Autodesk Inventor part; units mm, degrees
ref_plane "YZ Plane" through (0, 0, 0) normal (1, 0, 0) x (0, 1, 0)
ref_plane "XZ Plane" through (0, 0, 0) normal (0, 1, 0) x (-1, 0, 0)
ref_plane "XY Plane" through (0, 0, 0) normal (0, 0, 1) x (1, 0, 0)
sketch "Sketch1" plane through (0, 0, 0) normal (0, 0, 1) x (1, 0, 0)
  line L0 (-26.924, 25.4) -> (26.924, 25.4)
  line L1 (-26.924, 25.4) -> (-26.924, -19.05)
  line L2 (-14.224, -25.4) -> (-14.224, -20.32)
  line L3 (-15.494, -19.05) -> (-26.924, -19.05)
  line L4 (26.924, 25.4) -> (26.924, -19.05)
  line L5 (26.924, -19.05) -> (15.494, -19.05)
  line L6 (14.224, -20.32) -> (14.224, -25.4)
  line L7 (14.224, -25.4) -> (-14.224, -25.4)
  line L8 (-15.494, -19.05) -> (-14.224, -20.32)
  line L9 (14.224, -20.32) -> (15.494, -19.05)
  point P0 (0, 0)
  point P1 (-14.224, -19.05)
  point P2 (14.224, -19.05)
  dimension "d7" = 1.27
  dimension "d8" = 1.27
  dimension "d9" = 1.27
  dimension "d10" = 1.27
extrude "Extrusion1" add sketch "Sketch1" along normal blind 1.6
sketch "Sketch2" plane through (0, 0, 1.6) normal (0, 0, 1) x (1, 0, 0)
  line L0 (26.924, 25.4) -> (-26.924, 25.4)
  line L1 (-26.924, 25.4) -> (-26.924, 22.225)
  line L2 (-26.924, 25.4) -> (-26.924, -19.05)
  line L3 (-26.924, 22.225) -> (-23.749, 22.225)
  line L4 (26.924, 22.225) -> (23.749, 22.225)
  line L5 (14.224, -25.4) -> (-14.224, -25.4)
  line L6 (-14.224, -25.4) -> (-11.049, -25.4)
  line L7 (-11.049, -25.4) -> (-11.049, -22.225)
  line L8 (14.224, -25.4) -> (11.049, -25.4)
  line L9 (11.049, -25.4) -> (11.049, -22.225)
  line L10 (-26.924, -19.05) -> (-26.924, -10.922)
  line L11 (-26.924, -10.922) -> (-23.749, -10.922)
  point P0 (0, 0)
  dimension "d13" = 3.175
  dimension "d14" = 3.175
  dimension "d15" = 3.175
  dimension "d16" = 3.175
  dimension "d17" = 3.175
  dimension "d18" = 3.175
  dimension "d19" = 8.128
  dimension "d20" = 3.175
hole "Hole1" at (-23.749, 22.225, 1.6) at (23.749, 22.225, 1.6) at (-11.049, -22.225, 1.6) at (11.049, -22.225, 1.6) at (-23.749, -10.922, 1.6) direction (0, 0, -1) diameter 3.048 end through all
sketch "Sketch3" plane through (0, 0, 1.6) normal (0, 0, 1) x (1, 0, 0)
  line L0 (-26.924, 25.4) -> (26.924, 25.4)
  line L1 (0, 23.4) -> (8.5, 23.4)
  line L2 (8.5, 23.4) -> (8.5, 16.9)
  line L3 (8.5, 6.4) -> (-8.5, 6.4)
  line L4 (-8.5, 6.4) -> (-8.5, 12.9)
  line L5 (-8.5, 23.4) -> (0, 23.4)
  line L6 (-8.5, 23.4) -> (-8.5, 16.9)
  line L7 (-8.5, 12.9) -> (-10.5, 12.9)
  line L8 (-12.5, 14.9) -> (-12.5, 14.9)
  line L9 (-10.5, 16.9) -> (-8.5, 16.9)
  line L10 (-8.5, 16.9) -> (-8.5, 23.4)
  line L11 (8.5, 12.9) -> (10.5, 12.9)
  line L12 (12.5, 14.9) -> (12.5, 14.9)
  line L13 (10.5, 16.9) -> (8.5, 16.9)
  line L14 (8.5, 12.9) -> (8.5, 6.4)
  arc A0 (-10.5, 16.9) -> (-12.5, 14.9) centre (-10.5, 14.9) ccw
  arc A1 (-12.5, 14.9) -> (-10.5, 12.9) centre (-10.5, 14.9) ccw
  arc A2 (10.5, 12.9) -> (12.5, 14.9) centre (10.5, 14.9) ccw
  arc A3 (12.5, 14.9) -> (10.5, 16.9) centre (10.5, 14.9) ccw
  point P0 (0, 0)
  dimension "d35" = 2
extrude "Extrusion2" add sketch "Sketch3" along normal blind 8
sketch "Sketch4" plane through (0, 0, 9.6) normal (0, 0, 1) x (1, 0, 0)
  circle A0 centre (0, 14.9) radius 7.5
  point P0 (0, 0)
  dimension "d38" = 15
extrude "Extrusion3" add sketch "Sketch4" along normal blind 6.5
sketch "Sketch5" plane through (0, 14.9, 16.1) normal (0, 0, 1) x (1, 0, 0)
  circle A0 centre (0, 0) radius 6
  point P0 (0, -14.9)
  dimension "d41" = 12
extrude "Extrusion4" add sketch "Sketch5" along normal blind 5
sketch "Sketch6" plane through (0, 14.9, 21.1) normal (0, 0, 1) x (1, 0, 0)
  circle A0 centre (0, 0) radius 7
  point P0 (0, -14.9)
  dimension "d44" = 14
extrude "Extrusion5" add sketch "Sketch6" along normal blind 4
sketch "Sketch7" plane through (0, 14.9, 25.1) normal (0, 0, 1) x (1, 0, 0)
  circle A0 centre (0, 0) radius 5.5
  point P0 (0, -14.9)
  dimension "d47" = 11
extrude "Extrusion6" cut sketch "Sketch7" against normal blind 1
chamfer "Chamfer1" distance 1 angle 45 1 edges at (-5.5, 14.9, 24.1)
sketch "Sketch8" plane through (0, 0, 9.6) normal (0, 0, 1) x (1, 0, 0)
  line L0 (-8.5, 23.4) -> (8.5, 23.4)
  line L1 (0, 23.4) -> (1.25, 23.4)
  line L2 (1.25, 23.4) -> (1.25, 22.2951)
  line L3 (0, 23.4) -> (-1.25, 23.4)
  line L4 (-1.25, 23.4) -> (-1.25, 22.2951)
  arc A0 (-1.25, 22.2951) -> (1.25, 22.2951) centre (0, 14.9) ccw
  arc A1 (1.25, 22.2951) -> (-1.25, 22.2951) centre (0, 14.9) ccw
  point P0 (0, 0)
  dimension "d53" = 1.25
  dimension "d54" = 1.25
extrude "Extrusion7" add sketch "Sketch8" along normal up to surface (6.5 mm away) contours L0 L2 A1 L4
sketch "Sketch9" plane through (-8.5, 23.4, 1.6) normal (0, 1, 0) x (1, 0, 0)
  line L0 (7.25, -14.5) -> (9.75, -14.5)
  line L1 (8.5, -14.5) -> (8.5, -11.5)
  point P0 (8.5, 1.6)
  dimension "d57" = 3
hole "Hole2" at (0, 23.4, 13.1) direction (0, -1, 0) diameter 1.25 depth 3
sketch "Sketch10" plane through (0, 0, 9.6) normal (0, 0, 1) x (1, 0, 0)
  arc A0 (-10.5, 16.9) -> (-10.5, 12.9) centre (-10.5, 14.9) ccw
  arc A1 (10.5, 12.9) -> (10.5, 16.9) centre (10.5, 14.9) ccw
  point P0 (0, 0)
hole "Hole3" at (-10.5, 14.9, 9.6) at (10.5, 14.9, 9.6) direction (0, 0, -1) diameter 2 depth 8
sketch "Sketch11" plane through (0, 0, 0) normal (0, 0, -1) x (-1, 0, 0)
  line L0 (26.924, 25.4) -> (26.924, -19.05)
  line L1 (26.924, 25.4) -> (26.924, 24.4)
  line L2 (26.924, 24.4) -> (21.924, 24.4)
  line L3 (21.924, 24.4) -> (21.924, 4.4)
  line L4 (21.924, 4.4) -> (12.924, 4.4)
  line L5 (12.924, 4.4) -> (12.924, 24.4)
  line L6 (12.924, 24.4) -> (21.924, 24.4)
  point P0 (0, 0)
  dimension "d72" = 1
  dimension "d73" = 5
  dimension "d74" = 20
  dimension "d75" = 9
extrude "Extrusion8" add sketch "Sketch11" along normal blind 10
sketch "Sketch13" plane through (0, 0, 0) normal (0, 0, -1) x (-1, 0, 0)
  line L0 (-26.924, 25.4) -> (26.924, 25.4)
  line L1 (-26.924, 25.4) -> (-21.924, 25.4)
  line L2 (-21.924, 25.4) -> (-21.924, 17.9)
  line L3 (-21.924, 17.9) -> (-17.924, 17.9)
  line L4 (-17.924, 17.9) -> (-17.924, 9.9)
  line L5 (-17.924, 9.9) -> (-21.924, 9.9)
  line L6 (-21.924, 9.9) -> (-21.924, 17.9)
  point P0 (0, 0)
  dimension "d78" = 5
  dimension "d79" = 7.5
  dimension "d80" = 4
  dimension "d81" = 8
extrude "Extrusion9" add sketch "Sketch13" along normal blind 9.5
fillet "Fillet1" radius 0.5 4 edges at (21.924, 17.9, -4.75) (21.924, 9.9, -4.75) (17.924, 9.9, -4.75) (17.924, 17.9, -4.75)
sketch "Sketch14" plane through (0, 0, 1.6) normal (0, 0, 1) x (1, 0, 0)
  line L0 (-14.224, -25.4) -> (-14.224, -20.32)
  line L1 (-14.224, -25.4) -> (-1.524, -25.4)
  line L2 (14.224, -25.4) -> (-14.224, -25.4)
  line L3 (-1.524, -25.4) -> (-1.524, -21.4)
  line L4 (-1.524, -21.4) -> (1.976, -21.4)
  line L5 (1.976, -21.4) -> (1.976, -18.4)
  line L6 (1.976, -18.4) -> (-1.524, -18.4)
  line L7 (-1.524, -18.4) -> (-1.524, -21.4)
  point P0 (0, 0)
  dimension "d85" = 12.7
  dimension "d86" = 4
  dimension "d87" = 3.5
  dimension "d88" = 3
extrude "Extrusion10" add sketch "Sketch14" along normal blind 2
fillet "Fillet2" radius 0.25 10 edges at (1.25, 22.2951, 12.85) (-1.25, 22.2951, 12.85) (8.5, 23.4, 5.6) (8.5, 16.9, 5.6) (8.5, 6.4, 5.6) (-8.5, 23.4, 5.6) (-8.5, 16.9, 5.6) (-8.5, 12.9, 5.6) (8.5, 12.9, 5.6) (-8.5, 6.4, 5.6)
properties part number "PixyCMUcam5"
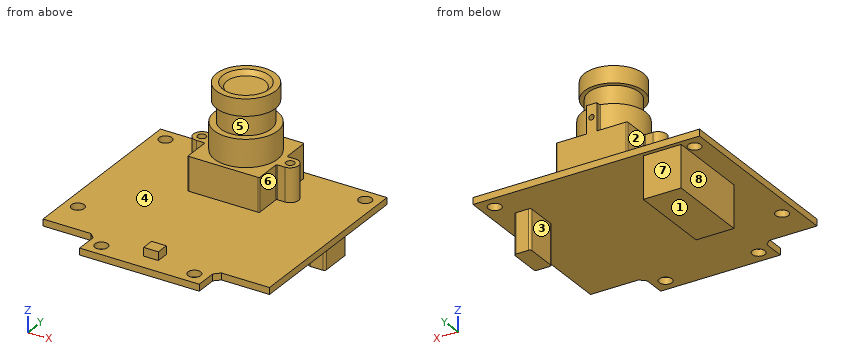
Can you work these out from the model? Positions are in its coordinate system, mm. Face numbers are marked on the shaded views. A direction names the side the tool comes from. Round coordinates to 2 decimals unless told otherwise and drop trailing zeros. Loops run counter-clockwise (first coordinate to the right, second up) from the corner with the lowest first, then second, coordinate; pieces in that order, holes last. Notation, with made-up numbers: M 32,83 L 86,83 A12 ccw 86,88 Z; hole C 0,73.25 d1. An arc over 180 degrees is marked long. Write item = value, one per line. Start each with the question number.
(1) I need wall thicknesses on line 1 along X through (y, z) = (14, 5); line 2 along Z through (x, y) = (-9, 12); line 3 along Z through (x, y) = (-5.5, 16). Which ranges of each line are inside material? Lowest first, please.
(2) Suppose I cut it at C-C on z = 8. Write out the boundary of the cut face in (x, y).
(3) Suppose I cut it at D-D on y = 1.5. Write out the boundary of the cut face in (x, z).
(4) I'm going to push flat-ended pins straight in: P1, Ø10, axis at y = 14.5, z = 15, coming from the -X side; P2, Ø0.9, axis at x = 9.5, z = 6.5, coming from the +Y side; P3, Ø17.5, axis at x = 0, y = 14.9, coming from the +Z side; P4, Ø7, axis at x = 0, y = 14, coming from the -Z side. Where does each tip first touch, or does it pass through?
(5) Which directions (+Z, -Z, +X, -X, +Y, -Y) give clear straight access to the entire face, cutting with the end or side of a thin tool? Please do the marked faces 4, 5, 6, 7 and 8.
(6) Suppose I cut it at B-B on z = -3.5. Write out the boundary of the cut face in (x, y), plus the area to 3 significant figures.
(7) If we mould it in two halves opening along X, with no side actions, what happens to the marked faces 1, 2 and 3? For each: released by +X, released by -X, zero draft, split by the parting line, or undercut.
(8) Suppose I cut it at A-A on z = 2.5. Write out the boundary of the cut face in (x, y), plus the area to 3 significant figures.
Answer block:
q1.line_1 = -12.29 to -10.94, -10.06 to 10.06, 10.94 to 12.29
q1.line_2 = 0 to 1.6
q1.line_3 = 0 to 25.1
q2.outline = M -10.5,12.9 L -8.75,12.9 A0.25 cw -8.5,12.65 L -8.5,6.65 A0.25 ccw -8.25,6.4 L 8.25,6.4 A0.25 ccw 8.5,6.65 L 8.5,12.65 A0.25 cw 8.75,12.9 L 10.5,12.9 A2 ccw 10.5,16.9 L 8.75,16.9 A0.25 cw 8.5,17.15 L 8.5,23.15 A0.25 ccw 8.25,23.4 L -8.25,23.4 A0.25 ccw -8.5,23.15 L -8.5,17.15 A0.25 cw -8.75,16.9 L -10.5,16.9 A2 ccw Z; hole C -10.5,14.9 d2; hole C 10.5,14.9 d2
q3.outline = M -26.92,0 L 26.92,0 L 26.92,1.6 L -26.92,1.6 Z
q4.P1 = -7.5
q4.P2 = 16.9
q4.P3 = 25.1
q4.P4 = 0
q5.face_4 = +Z
q5.face_5 = none
q5.face_6 = +Z, +X, -Y
q5.face_7 = -Z, +X, -X, +Y
q5.face_8 = -Z, -X, +Y, -Y
q6.outline = M -21.92,4.4 L -12.92,4.4 L -12.92,24.4 L -21.92,24.4 Z; M 17.92,10.4 A0.5 ccw 18.42,9.9 L 21.42,9.9 A0.5 ccw 21.92,10.4 L 21.92,17.4 A0.5 ccw 21.42,17.9 L 18.42,17.9 A0.5 ccw 17.92,17.4 Z
q6.area = 212 mm²
q7.face_1 = zero draft
q7.face_2 = released by -X
q7.face_3 = undercut
q8.outline = M -10.5,12.9 L -8.75,12.9 A0.25 cw -8.5,12.65 L -8.5,6.65 A0.25 ccw -8.25,6.4 L 8.25,6.4 A0.25 ccw 8.5,6.65 L 8.5,12.65 A0.25 cw 8.75,12.9 L 10.5,12.9 A2 ccw 10.5,16.9 L 8.75,16.9 A0.25 cw 8.5,17.15 L 8.5,23.15 A0.25 ccw 8.25,23.4 L -8.25,23.4 A0.25 ccw -8.5,23.15 L -8.5,17.15 A0.25 cw -8.75,16.9 L -10.5,16.9 A2 ccw Z; M -1.52,-21.4 L 1.98,-21.4 L 1.98,-18.4 L -1.52,-18.4 Z; hole C -10.5,14.9 d2; hole C 10.5,14.9 d2
q8.area = 322 mm²
